The listing builds one solid part. Answer for the finished solid, in the listing's coordinates (mm). A direction names the side the tool comes from. Coordinates: 2 decimals unless noted, no trailing zeros. Order: outer loops, then holes, each group sorted by start corner. A loop starts at its lowest first (then second) coordinate and runs counter-clockwise, first axis right, second up. Notation, with made-up numbers: (47, -16) -> (102, -16) arc R12 ccw to (102, 5) -> close; hole circle Ø3 at (59, 45). An arc over 180 degrees is marked (long way). Return JSON: item names as keys, results as strings.
from build123d import *

# Parameters (mm, degrees)
SKETCH_1_W            = 90
SKETCH_1_H            = 120
SKETCH_1_R            = 2
SKETCH_1_R_2          = 1.6
EXTRUDE_1_DEPTH       = 5
FILLET_1_R            = 8
F_3_2_PCD16_R         = 1.6
CUT_EXTRUDE_3_2_DEPTH = 10
XRU1008_6_1_2_R       = 3
XRU1008_6_1_DEPTH     = 1


with BuildPart() as part:
    # Sketch 1 → Extrude 1 (new body)
    with BuildSketch(Plane.XY):
        with Locations((45, -60)):
            Rectangle(SKETCH_1_W, SKETCH_1_H)
        with Locations((79, -45)):
            Circle(SKETCH_1_R, mode=Mode.SUBTRACT)
        with Locations((79, -75)):
            Circle(SKETCH_1_R, mode=Mode.SUBTRACT)
        with Locations((85, -102.5)):
            Circle(SKETCH_1_R_2, mode=Mode.SUBTRACT)
        with Locations((75, -102.5)):
            Circle(SKETCH_1_R_2, mode=Mode.SUBTRACT)
        with Locations((65, -102.5)):
            Circle(SKETCH_1_R_2, mode=Mode.SUBTRACT)
        with Locations((55, -102.5)):
            Circle(SKETCH_1_R_2, mode=Mode.SUBTRACT)
        with Locations((45, -102.5)):
            Circle(SKETCH_1_R_2, mode=Mode.SUBTRACT)
        with Locations((85, -17.5)):
            Circle(SKETCH_1_R_2, mode=Mode.SUBTRACT)
        with Locations((75, -17.5)):
            Circle(SKETCH_1_R_2, mode=Mode.SUBTRACT)
        with Locations((65, -17.5)):
            Circle(SKETCH_1_R_2, mode=Mode.SUBTRACT)
        with Locations((55, -17.5)):
            Circle(SKETCH_1_R_2, mode=Mode.SUBTRACT)
        with Locations((45, -17.5)):
            Circle(SKETCH_1_R_2, mode=Mode.SUBTRACT)
        with Locations((35, -102.5)):
            Circle(SKETCH_1_R_2, mode=Mode.SUBTRACT)
        with Locations((25, -102.5)):
            Circle(SKETCH_1_R_2, mode=Mode.SUBTRACT)
        with Locations((15, -102.5)):
            Circle(SKETCH_1_R_2, mode=Mode.SUBTRACT)
        with Locations((35, -17.5)):
            Circle(SKETCH_1_R_2, mode=Mode.SUBTRACT)
        with Locations((25, -17.5)):
            Circle(SKETCH_1_R_2, mode=Mode.SUBTRACT)
        with Locations((15, -17.5)):
            Circle(SKETCH_1_R_2, mode=Mode.SUBTRACT)
        with Locations((8, -102.5)):
            Circle(SKETCH_1_R_2, mode=Mode.SUBTRACT)
        with Locations((8, -17.5)):
            Circle(SKETCH_1_R_2, mode=Mode.SUBTRACT)
        Polygon((50.616580754, -42.2), (47.383419246, -42.2), (45.766838493, -45), (47.383419246, -47.8), (50.616580754, -47.8), (52.233161507, -45), align=None, mode=Mode.SUBTRACT)
        Polygon((50.616580754, -72.2), (47.383419246, -72.2), (45.766838493, -75), (47.383419246, -77.8), (50.616580754, -77.8), (52.233161507, -75), align=None, mode=Mode.SUBTRACT)
    extrude(amount=EXTRUDE_1_DEPTH)

    # Fillet 1
    fillet_1_edges = [part.edges().sort_by_distance(p)[0] for p in [
        (0, 0, 2.5),
        (90, 0, 2.5),
        (90, -120, 2.5),
        (0, -120, 2.5),
    ]]
    fillet(fillet_1_edges, radius=FILLET_1_R)

    # 3.2_PCD16 → Cut-Extrude 3.2 (cut)
    with BuildSketch(Plane(origin=(0, 0, 0), x_dir=(-1, 0, 0), z_dir=(0, 0, -1))):
        with Locations((-46.156854249, -54.343145751)):
            Circle(F_3_2_PCD16_R)
        with Locations((-34.843145751, -54.343145751)):
            Circle(F_3_2_PCD16_R)
        with Locations((-34.843145751, -65.656854249)):
            Circle(F_3_2_PCD16_R)
        with Locations((-46.156854249, -65.656854249)):
            Circle(F_3_2_PCD16_R)
    extrude(amount=-CUT_EXTRUDE_3_2_DEPTH, mode=Mode.SUBTRACT)

    # XRU1008__6___1 2 → XRU1008__6___1 (cut)
    with BuildSketch(Plane.XY.offset(5)):
        with Locations((46.156854249, -54.343145751)):
            Circle(XRU1008_6_1_2_R)
        with Locations((34.843145751, -54.343145751)):
            Circle(XRU1008_6_1_2_R)
        with Locations((34.843145751, -65.656854249)):
            Circle(XRU1008_6_1_2_R)
        with Locations((46.156854249, -65.656854249)):
            Circle(XRU1008_6_1_2_R)
    extrude(amount=-XRU1008_6_1_DEPTH, mode=Mode.SUBTRACT)


solid = part.part
1. Consider line 1 (Y direction, x = 79, z = 3.65); line 2 (Y direction, x = 8, z = 1.25). Determine where each line is inside the solid, lowest interval first. Write a range as from..to.
Answer block:
{"line 1": "y = -120..-77, -73..-47, -43..0", "line 2": "y = -120..-104.1, -100.9..-19.1, -15.9..0"}
2. The part is cut by section A-A on x = 79. Give the vertices of the cut face in (y, z), and give its area (3 significant figures).
Answer block:
{"outline": "(-120, 0) -> (-77, 0) -> (-77, 5) -> (-120, 5) -> close; (-73, 0) -> (-47, 0) -> (-47, 5) -> (-73, 5) -> close; (-43, 0) -> (0, 0) -> (0, 5) -> (-43, 5) -> close", "area": "560 mm2"}
3. Each of these flat-tipped pins is pushed along its axis until it touches: pin 1 Ø2.5 at (x, y) = (8, -17.5) entering from +Z; pin 2 Ø3.5 at (x, y) = (34.84, -65.66) entering from +Z. Where does it stop, or does it pass through?
Answer block:
{"pin 1": "passes through", "pin 2": "stops at z = 4"}
4. For faces 1 (the face through (87.594, -2.281, 2.535)), 2 (the face through (51.436, -73.62, 2.465)), 3 (the face through (47.77, -51.814, 4.507)), determine the directions among +Z, -Z, +X, -X, +Y, -Y from which every point of the face is accessible in a straight line to the end or side of a thin tool.
Answer block:
{"face 1": "+Z, -Z, +X, +Y", "face 2": "+Z, -Z", "face 3": "+Z"}
5. The part is cut by section C-C on x = 35. Give the vertices of the cut face in (y, z).
Answer block:
{"outline": "(-120, 0) -> (-104.1, 0) -> (-104.1, 5) -> (-120, 5) -> close; (-100.9, 0) -> (-67.25, 0) -> (-67.25, 4) -> (-68.65, 4) -> (-68.65, 5) -> (-100.9, 5) -> close; (-64.06, 0) -> (-55.94, 0) -> (-55.94, 4) -> (-57.34, 4) -> (-57.34, 5) -> (-62.66, 5) -> (-62.66, 4) -> (-64.06, 4) -> close; (-52.75, 0) -> (-19.1, 0) -> (-19.1, 5) -> (-51.35, 5) -> (-51.35, 4) -> (-52.75, 4) -> close; (-15.9, 0) -> (0, 0) -> (0, 5) -> (-15.9, 5) -> close"}
6. The part is cut by section B-B on y = -102.5. Give the number of separate pieces and of enclosed holes in the cut face, and give its area (3 significant figures).
Answer block:
{"separate pieces": "10", "enclosed holes": "0", "area": "306 mm2"}
7. Determine the mould class of faces 4 (the face through (34.105, -67.076, 1.972)), 5 (the face through (44, -59, 5)), 6 (the face through (87.594, -117.719, 2.535)), 7 (the face through (36, -67, 4)) for opening direction X: pulls with the +X half, pulls with the -X half, needs draft (parallel to the pull), parting line crosses it, or undercut.
Answer block:
{"face 4": "undercut", "face 5": "needs draft", "face 6": "pulls with the +X half", "face 7": "undercut"}
8. The part is cut by section D-D on x = 25. Give the vertices of the cut face in (y, z), and give its area (3 significant figures).
Answer block:
{"outline": "(-120, 0) -> (-104.1, 0) -> (-104.1, 5) -> (-120, 5) -> close; (-100.9, 0) -> (-19.1, 0) -> (-19.1, 5) -> (-100.9, 5) -> close; (-15.9, 0) -> (0, 0) -> (0, 5) -> (-15.9, 5) -> close", "area": "568 mm2"}
